Autodesk Inventor part; units mm, degrees
ref_plane "YZ Plane" through (0, 0, 0) normal (1, 0, 0) x (0, 1, 0)
ref_plane "XZ Plane" through (0, 0, 0) normal (0, 1, 0) x (-1, 0, 0)
ref_plane "XY Plane" through (0, 0, 0) normal (0, 0, 1) x (1, 0, 0)
sketch "Skizze1" plane through (0, 0, 0) normal (0, 0, 1) x (1, 0, 0)
  line L0 (0, -28.5) -> (0, 27.5)
  line L1 (-71.9, 0) -> (35.9, 0)
  circle A0 centre (-15.5, 15.5) radius 1.55
  circle A1 centre (15.5, 15.5) radius 1.55
  circle A2 centre (-15.5, -15.5) radius 1.55
  circle A3 centre (15.5, -15.5) radius 1.55
  circle A4 centre (-16.5, 0) radius 11
  circle A5 centre (0, 0) radius 5.5
  circle A6 centre (-16.5, 0) radius 4
  arc A7 (-16.5, -7.5) -> (-16.5, 7.5) centre (-16.5, 0) ccw
  line L2 (-16.5, 7.5) -> (-36.5, 7.5)
  line L3 (-36.5, 7.5) -> (-56.5, 7.5)
  line L4 (-56.5, 7.5) -> (-56.5, -7.5)
  line L5 (-56.5, -7.5) -> (-16.5, -7.5)
  circle A8 centre (15.5, 15.5) radius 4
  circle A9 centre (15.5, -15.5) radius 5
  circle A10 centre (-15.5, 15.5) radius 4
  circle A11 centre (-15.5, -15.5) radius 4
  line L6 (15.5, 11.5) -> (-15.5, 11.5)
  line L7 (15.5, 19.5) -> (-15.5, 19.5)
  line L8 (-15.5, 19.5) -> (-50.5, 19.5)
  line L9 (-50.5, 19.5) -> (-50.5, 7.5)
  line L10 (-15.5, 11.5) -> (-30.5, 11.5)
  line L11 (-30.5, 11.5) -> (-30.5, 7.5)
  dimension "d0" = 3.1
  dimension "d1" = 15.5
  dimension "d2" = 15.5
  dimension "d3" = 22
  dimension "d4" = 16.5
  dimension "d5" = 11
  dimension "d6" = 8
  dimension "d7" = 15
  dimension "d10" = 15
  dimension "d11" = 40
  dimension "d17" = 8
  dimension "d18" = 10
  dimension "d19" = 8
  dimension "d20" = 8
  dimension "d22" = 35
  dimension "d23" = 15
extrude "Extrusion3" add sketch "Skizze1" along normal blind 5 contours L6 A10 L7 L0 | L0 L7 A8 L6 | L2 L3 L9 L8 A10 L10 L11 | A8 | A10
sketch "Skizze3" plane through (0, 0, 5) normal (0, 0, 1) x (1, 0, 0)
  circle A0 centre (0, 0) radius 12
  circle A1 centre (-13.5, -33.5) radius 2.75
  circle A2 centre (13.5, -33.5) radius 2.75
  circle A3 centre (-15.5, -15.5) radius 1.75
  circle A4 centre (15.5, -15.5) radius 1.75
  circle A5 centre (-15.5, 15.5) radius 1.75
  circle A6 centre (15.5, 15.5) radius 1.75
  line L0 (19.5, -43.5) -> (21.5, -41.5)
  line L1 (21.5, -41.5) -> (21.5, 19.5)
  line L2 (21.5, 19.5) -> (19.5, 21.5)
  line L3 (19.5, 21.5) -> (-19.5, 21.5)
  line L4 (-19.5, 21.5) -> (-21.5, 19.5)
  line L5 (-21.5, 19.5) -> (-21.5, -41.5)
  line L6 (-21.5, -41.5) -> (-19.5, -43.5)
  line L7 (-19.5, -43.5) -> (19.5, -43.5)
  line L8 (-30.5, 11.5) -> (15.5, 11.5)
  line L9 (3.4278, 11.5) -> (-3.4278, 11.5)
  point P0 (0, 0)
extrude "Extrusion4" cut sketch "Skizze3" against normal blind 5 contours L8 A0 picked at (0.3856, 11.648)
fillet "Rundung1" radius 2 1 edges at (-50.5, 19.5, 2.5)
properties part number "Drückbrücke" material "ABS-Kunststoff"
Here's how the part is built. I have some questions about the finished solid (model axes, mm). A direction names the side the tool comes from. Give positions to 0.01 mm unless a question says otherwise; leave off trailing zeros. Write each loop counter-clockwise with the first axis right and the second up, starting at its lowest first coordinate (ties: lowest second). Pieces come first, ordered by that corner, then holes. Notation, with made-up numbers: (-20.5, 7) -> (-11.5, 7) arc R25 cw to (-11.5, 27) -> close; hole circle Ø1 at (-29.75, 89.25). An arc over 180 degrees is marked (long way). Use one line per item in the form item = value. Start each with the question number.
1. Thinking about a two-plate mould opening in X: for faces 1 (the face through (0, 12, 3)), 2 (the face through (10, 11.5, 2)), 3 (the face through (-50.5, 13, 2)), which applies, +X half, -X half, draft (parallel to the pull), parting line (faces both ways), or undercut?
2. On a 3-axis mill with a long thin cutter (end or side, diameter ignored), from which of +Z, -Z, +X, -X, +Y, -Y can I reach the whole of each face in a straight line? I mean faces 4 (the face through (-16.64, 14.45, 2.46)), 5 (the face through (-30.5, 10, 2)). Say none if no direction works.
3. If I drill on L1, parallel to Y at x = -15.5, z = 1.3; L2, parallel to X at y = 15, z = 2.4; L3, parallel to Y at x = -29, z = 1.35, over which ranges is the centre line in solid material (lowest first)?
4. Imagine slicing it at A-A on y = 15.5. List the corners of the cut face in (x, z) for me.
5. Imagine slicing it at C-C on z = 4.25. List the corners of the cut face in (x, y) for me, plus the area to 3 significant figures.
6. Imagine slicing it at D-D on y = 10.5. List the corners of the cut face in (x, z) for me.
7. Will these pins go through, and if not, where does the flat tip stop? pin 1 Ø3 at (x, y) = (-15.5, 15.5) entering from -Z; pin 2 Ø2 at (y, z) = (9.5, 2.5) entering from +X.
8. Imagine slicing it at B-B on x = -15.5. List the corners of the cut face in (y, z) for me.
Entries:
q1.face_1 = undercut
q1.face_2 = draft
q1.face_3 = -X half
q2.face_4 = +Z, -Z
q2.face_5 = +Z, -Z, +X, -Y
q3.L1 = 11.5 to 13.95, 17.05 to 19.5
q3.L2 = -50.5 to -16.97, -14.03 to 14.03, 16.97 to 19.47
q3.L3 = 11.5 to 19.5
q4.outline = (-50.5, 0) -> (-17.05, 0) -> (-17.05, 5) -> (-50.5, 5) -> close; (-13.95, 0) -> (13.95, 0) -> (13.95, 5) -> (-13.95, 5) -> close; (17.05, 0) -> (19.5, 0) -> (19.5, 5) -> (17.05, 5) -> close
q5.outline = (-50.5, 7.5) -> (-30.5, 7.5) -> (-30.5, 11.5) -> (-3.43, 11.5) arc R12 cw to (3.43, 11.5) -> (15.5, 11.5) arc R4 ccw to (15.5, 19.5) -> (-48.5, 19.5) arc R2 ccw to (-50.5, 17.5) -> close; hole circle Ø3.1 at (-15.5, 15.5); hole circle Ø3.1 at (15.5, 15.5)
q5.area = 615 mm²
q6.outline = (-50.5, 0) -> (-30.5, 0) -> (-30.5, 5) -> (-50.5, 5) -> close
q7.pin_1 = through
q7.pin_2 = -30.5
q8.outline = (11.5, 0) -> (13.95, 0) -> (13.95, 5) -> (11.5, 5) -> close; (17.05, 0) -> (19.5, 0) -> (19.5, 5) -> (17.05, 5) -> close
